```python
from build123d import *

# Parameters (mm, degrees)
SKETCH3_W           = 120
SKETCH3_H           = 17
BOSS_EXTRUDE1_DEPTH = 86
SKETCH5_W           = 120
SKETCH5_H           = 75
BOSS_EXTRUDE2_DEPTH = 16
BOSS_EXTRUDE3_DEPTH = 25
SKETCH11_R          = 8
CUT_EXTRUDE1_DEPTH  = 25
FILLET2_R           = 25
FILLET3_R           = 25
FILLET11_R          = 8
BOSS_EXTRUDE4_DEPTH = 65
CUT_EXTRUDE2_DEPTH  = 55
FILLET15_R          = 8
SKETCH16_R          = 10
CUT_EXTRUDE3_DEPTH  = 55
SKETCH17_R          = 10
CUT_EXTRUDE4_DEPTH  = 55


with BuildPart() as part:
    # Sketch3 → Boss-Extrude1 (new body)
    with BuildSketch(Plane(origin=(0, 0, 0), x_dir=(0, 0, -1), z_dir=(1, 0, 0))):
        with Locations((60, 8.5)):
            Rectangle(SKETCH3_W, SKETCH3_H)
    extrude(amount=BOSS_EXTRUDE1_DEPTH)

    # Sketch5 → Boss-Extrude2 (add)
    with BuildSketch(Plane(origin=(86, 0, 0), x_dir=(0, 0, -1), z_dir=(1, 0, 0))):
        with Locations((60, 37.5)):
            Rectangle(SKETCH5_W, SKETCH5_H)
    extrude(amount=-BOSS_EXTRUDE2_DEPTH)

    # Sketch7 → Boss-Extrude3 (add)
    with BuildSketch(Plane(origin=(0, 75, 0), x_dir=(1, 0, 0), z_dir=(0, 1, 0))):
        with BuildLine():
            Line((138.227979275, 90.466321244), (86, 120))
            Line((86, 120), (86, 60))
            Line((86, 60), (86, 0))
            Line((86, 0), (138.227979275, 29.533678756))
            ThreePointArc((138.227979275, 29.533678756), (156, 60), (138.227979275, 90.466321244))
        make_face()
    extrude(amount=-BOSS_EXTRUDE3_DEPTH)

    # Sketch11 → Cut-Extrude1 (cut)
    with BuildSketch(Plane(origin=(0, 75, 0), x_dir=(1, 0, 0), z_dir=(0, 1, 0))):
        with Locations(Location((121, 60, 0), (0, 0, 270))):
            Circle(SKETCH11_R)
    extrude(amount=-CUT_EXTRUDE1_DEPTH, mode=Mode.SUBTRACT)

    # Fillet2
    fillet2_edges = [part.edges().sort_by_distance(p)[0] for p in [
        (0, 8.5, 0),
    ]]
    fillet(fillet2_edges, radius=FILLET2_R)

    # Fillet3
    fillet3_edges = [part.edges().sort_by_distance(p)[0] for p in [
        (0, 8.5, -120),
    ]]
    fillet(fillet3_edges, radius=FILLET3_R)

    # Fillet11
    fillet11_edges = [part.edges().sort_by_distance(p)[0] for p in [
        (70, 17, -60),
    ]]
    fillet(fillet11_edges, radius=FILLET11_R)

    # Sketch14 → Boss-Extrude4 (add)
    with BuildSketch(Plane.XY):
        Polygon((70, 75), (0, 17), (70, 17), align=None)
    extrude(amount=-BOSS_EXTRUDE4_DEPTH)

    # Sketch15 → Cut-Extrude2 (cut)
    with BuildSketch(Plane.XY):
        Polygon((0, 17), (70, 75), (70, 17), align=None)
    extrude(amount=-CUT_EXTRUDE2_DEPTH, mode=Mode.SUBTRACT)

    # Fillet15
    fillet15_edges = [part.edges().sort_by_distance(p)[0] for p in [
        (70, 17, -27.5),
    ]]
    fillet(fillet15_edges, radius=FILLET15_R)

    # Sketch16 → Cut-Extrude3 (cut)
    with BuildSketch(Plane(origin=(0, 17, 0), x_dir=(1, 0, 0), z_dir=(0, 1, 0))):
        with Locations(Location((25, 95, 0), (0, 0, 270))):
            Circle(SKETCH16_R)
    extrude(amount=-CUT_EXTRUDE3_DEPTH, mode=Mode.SUBTRACT)

    # Sketch17 → Cut-Extrude4 (cut)
    with BuildSketch(Plane(origin=(0, 17, 0), x_dir=(1, 0, 0), z_dir=(0, 1, 0))):
        with Locations(Location((25, 25, 0), (0, 0, 180))):
            Circle(SKETCH17_R)
    extrude(amount=-CUT_EXTRUDE4_DEPTH, mode=Mode.SUBTRACT)


solid = part.part
```
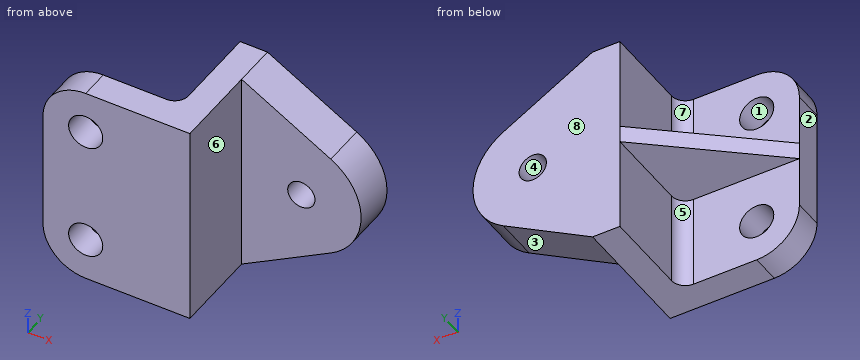
CAD build for the part. Positions are in the model's coordinates, mm. Face numbers are marked on the shaded views. A direction names the side the tool comes from. Round coordinates to 2 decimals unless told otherwise and drop trailing zeros. Order: outer loops, then holes, each group sorted by start corner. A loop starts at its lowest first (then second) coordinate and runs counter-clockwise, first axis right, second up.
Item 1: Mould opens along Z. For the marked faces 1, 2, 3 and 4 say: pulls with the +Z half, pulls with the -Z half, needs draft (parallel to the pull), parting line crosses it, or undercut.
Item 2: Saw through at D-D on x = 56. Write the cut outline in (y, z), then the cut area to 3 significant figures.
Item 3: Pin check, flat tips, straight feed: pin 1 (23 mm diameter, centred on x = 25, z = -95, fed in from +Y); pin 2 (6 mm diameter, centred on x = 139.5, y = 50, fed in from -Z); pin 3 (2 mm diameter, centred on x = 126.5, z = -20, fed in from -Y); pin 4 (3 mm diameter, centred on x = 48.5, y = 54.5, fed in from +Z). Stop position of each tip, or through.
Item 4: Saw through at B-B on x = 121. Write the cut outline in (y, z), then the cut area to 3 significant figures.
Item 5: Saw through at C-C on y = 54.5. Write the cut outline in (x, z), then the cut area to 3 significant figures.
Item 6: Probe line 1 along X through (y, z) = (10, -95); line 2 along Y through (x, z) = (31, -41); line 3 along X through (y, z) = (5, -39). List the from-to ranges inside material, lowest first.
Item 7: Saw through at A-A on z = -60. Write the cut outline in (x, y).
Item 8: Tool access for the marked faces 5, 6, 7 and 8: list every direction of +Z, -Z, +X, -X, +Y, -Y with a clear straight run to the whole face (end or side of a thin tool).
Reported:
1. face 1: undercut
1. face 2: needs draft
1. face 3: pulls with the -Z half
1. face 4: undercut
2. outline: (0, -120) - (17, -120) - (17, -65) - (63.4, -65) - (63.4, -55) - (17, -55) - (17, 0) - (0, 0) - close
2. area: 2,500 mm2
3. pin 1: stops at y = 17
3. pin 2: stops at z = -91.44
3. pin 3: passes through
3. pin 4: stops at z = -55
4. outline: (50, -100.21) - (75, -100.21) - (75, -68) - (50, -68) - close; (50, -52) - (75, -52) - (75, -19.79) - (50, -19.79) - close
4. area: 1,610 mm2
5. outline: (45.26, -65) - (70, -65) - (70, -120) - (86, -120) - (138.23, -90.47) arc R35 ccw to (138.23, -29.53) - (86, 0) - (70, 0) - (70, -55) - (45.26, -55) - close; hole circle Ø16 at (121, -60)
5. area: 7,460 mm2
6. line 1: x = 0 to 15, 35 to 86
6. line 2: y = 0 to 17
6. line 3: x = 0 to 86
7. outline: (0, 0) - (86, 0) - (86, 50) - (113, 50) - (113, 75) - (70, 75) - (0, 17) - close; (129, 50) - (156, 50) - (156, 75) - (129, 75) - close
8. face 5: -Z, -X, +Y
8. face 6: +Z, -Z, +X, -Y
8. face 7: +Z, -X, +Y
8. face 8: +Z, -Z, +X, -X, +Y
